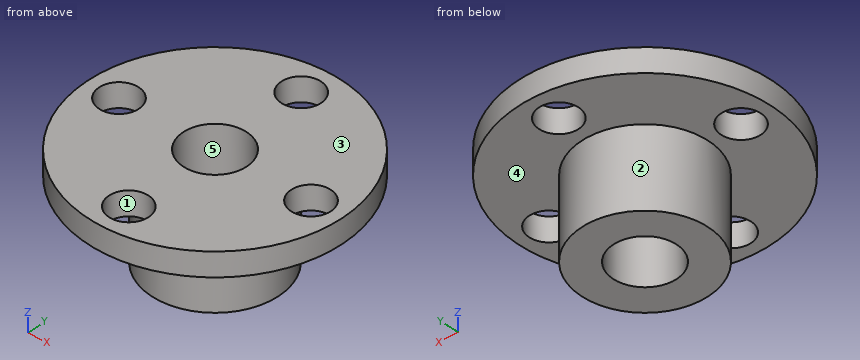
Autodesk Inventor part; units mm, degrees
ref_plane "YZ Plane" through (0, 0, 0) normal (1, 0, 0) x (0, 1, 0)
ref_plane "XZ Plane" through (0, 0, 0) normal (0, 1, 0) x (-1, 0, 0)
ref_plane "XY Plane" through (0, 0, 0) normal (0, 0, 1) x (1, 0, 0)
sketch "Sketch1" plane through (0, 0, 0) normal (0, 0, 1) x (1, 0, 0)
  circle A0 centre (0, 0) radius 4
  circle A1 centre (0, 0) radius 8
  dimension "d0" = 8
  dimension "d1" = 16
extrude "Extrusion1" add sketch "Sketch1" along normal blind 13
sketch "Sketch2" plane through (0, 0, 13) normal (0, 0, 1) x (1, 0, 0)
  circle A0 centre (0, 0) radius 16
  circle A1 centre (0, 0) radius 8
  dimension "d4" = 32
extrude "Extrusion2" add sketch "Sketch2" against normal blind 3
sketch "Sketch3" plane through (0, 0, 13) normal (0, 0, 1) x (1, 0, 0)
  circle A0 centre (12, 0) radius 2.5
  circle A1 centre (0, 12) radius 2.5
  circle A2 centre (-12, 0) radius 2.5
  circle A3 centre (0, -12) radius 2.5
  point P0 (0, 0)
  dimension "d7" = 5
  dimension "d8" = 12
  dimension "d11" = 360
extrude "Extrusion3" cut sketch "Sketch3" against normal through all
properties part number "8mm Mounting Hub" material "Steel, Mild"
Can you work these out from the model? Positions are in its coordinate system, mm. Face numbers are marked on the shaded views. A direction names the side the tool comes from. Give positions to 0.01 mm unless a question says otherwise; leave off trailing zeros. Write each loop counter-clockwise with the first axis right and the second up, starting at its lowest first coordinate (ties: lowest second). Pieces come first, ordered by that corner, then holes. Notation, with made-up numbers: (46.5, 54) - (77.5, 54) arc R23 ccw to (77.5, 86) - close; hole circle Ø1 at (-18, 46.5). An arc over 180 degrees is marked (long way). Write item = value, one per line. Start each with the question number.
1. Thinking about a two-plate mould opening in X: for the marked faces 1, 2 and 3, which applies, released by +X, released by -X, zero draft, split by the parting line, or undercut?
2. On a 3-axis mill with a long thin cutter (end or side, diameter ignored), from which of +Z, -Z, +X, -X, +Y, -Y can I reach the whole of each face in a straight line? I mean the marked faces 4 and 5. Say none if no direction works.
3. Imagine slicing it at A-A (y = 0). Please give me the cut outline in (x, z), and give its area (3 significant figures).
4. Imagine slicing it at D-D (x = -12). Please give me the cut outline in (y, z), and give its area (3 significant figures).
5. Please list where these lines run through material, in increasing order: line 1 (Y direction, x = 0, z = 12.1); line 2 (Y direction, x = 0, z = 3.75); line 3 (X direction, y = 10.5, z = 12).
6. For pin 1 (2 mm diameter, centred on y = -5, z = 2, fed in from +X); pin 2 (3 mm diameter, centred on x = 0, y = 12, fed in from +Z); pin 3 (1.5 mm diameter, centred on x = -11.5, y = -8.5, fed in from -Z); pin 4 (3 mm diameter, centred on x = -6.5, z = 9.5, fed in from +Y), each with a flat end and sliding along its axis, tell me the tip position at first contact or that it passes through.
7. Imagine slicing it at C-C (y = -13). Please give me the cut outline in (x, z), and give its area (3 significant figures).
Worked answers:
q1.face_1 = undercut
q1.face_2 = split by the parting line
q1.face_3 = zero draft
q2.face_4 = -Z
q2.face_5 = +Z, -Z
q3.outline = (-16, 10) - (-14.5, 10) - (-14.5, 13) - (-16, 13) - close; (-9.5, 10) - (-8, 10) - (-8, 0) - (-4, 0) - (-4, 13) - (-9.5, 13) - close; (4, 0) - (8, 0) - (8, 10) - (9.5, 10) - (9.5, 13) - (4, 13) - close; (14.5, 10) - (16, 10) - (16, 13) - (14.5, 13) - close
q3.area = 122 mm2
q4.outline = (-10.58, 10) - (-2.5, 10) - (-2.5, 13) - (-10.58, 13) - close; (2.5, 10) - (10.58, 10) - (10.58, 13) - (2.5, 13) - close
q4.area = 48.5 mm2
q5.line_1 = -16 to -14.5, -9.5 to -4, 4 to 9.5, 14.5 to 16
q5.line_2 = -8 to -4, 4 to 8
q5.line_3 = -12.07 to -2, 2 to 12.07
q6.pin_1 = 6.93
q6.pin_2 = through
q6.pin_3 = 10
q6.pin_4 = 15.17
q7.outline = (-9.33, 10) - (-2.29, 10) - (-2.29, 13) - (-9.33, 13) - close; (2.29, 10) - (9.33, 10) - (9.33, 13) - (2.29, 13) - close
q7.area = 42.2 mm2
